```python
from build123d import *

# Parameters (mm, degrees)
F0_R     = 1.5875
F1_DEPTH = 12.7
F2_W     = 4.18922
F2_H     = 3.175
F3_DEPTH = 1.5875
F4_W     = 3.647596
F4_H     = 5.093468
F4_H_2   = 3.670235
F5_DEPTH = 25.4


with BuildPart() as f1:
    # F0 (on Right) → F1 (new body, symmetric)
    with BuildSketch(Plane.YZ):
        Circle(F0_R)
    extrude(amount=F1_DEPTH, both=True)

    # F2 (on face) → F3 (join)
    with BuildSketch(Plane(origin=(-12.7, 0, 0), x_dir=(0, -1, 0), z_dir=(-1, 0, 0))):
        with Locations((-2.09461, 0)):
            Rectangle(F2_W, F2_H)
    extrude(amount=F3_DEPTH)

    # F4 (on face) → F5 (cut)
    with BuildSketch(Plane.XY.offset(1.5875)):
        with BuildLine():
            ThreePointArc((10.658555, 1.5875), (9.327825, -0.125735), (7.724933, -1.5875))
            Line((7.724933, -1.5875), (12.7, -1.5875))
            Line((12.7, -1.5875), (12.7, 1.5875))
            Line((12.7, 1.5875), (10.658555, 1.5875))
        make_face()
        with Locations((-13.995515, -0.959234)):
            Rectangle(F4_W, F4_H)
        with Locations((-13.995515, 3.422617)):
            Rectangle(F4_W, F4_H_2)
    extrude(amount=-F5_DEPTH, mode=Mode.SUBTRACT)


solid = f1.part
```
Can you work these out from the model? Positions are in its coordinate system, mm. Give positions to 0.01 mm unless a question says otherwise; leave off trailing zeros. Loops run counter-clockwise (first coordinate to the right, second up) from the corner with the lowest first, then second, coordinate; pieces in that order, holes last. Notation, with made-up numbers: M 69.5,81.25 L 76.5,81.25 A15 cw 76.5,104.25 Z; hole C 3,65.5 d3. An arc over 180 degrees is marked long. Use CSV: the item, a comma, the result in double quotes. Start each with the question number.
1. Imagine slicing it at A-A, the plane x = 0.25. Write out the boundary of the cut face in (y, z) (1 decimal), plus the area to 3 significant figures.
2. If I drill on L1, parallel to Y at x = -3.5, z = 0.1; L2, parallel to Y at x = 6.75, z = -1.1; L3, parallel to Z at x = -10.25, y = 0.6, over which ranges is the centre line in solid material (lowest first)?
3. Imagine slicing it at B-B, the plane z = 0. Write out the boundary of the cut face in (x, y), plus the area to 3 significant figures.
4. Imagine slicing it at C-C, the plane y = -0.4. Write out the boundary of the cut face in (x, z).
5. For P1, Ø1.5, axis at x = -2, y = 1, coming from the +Z side; P2, Ø1, axis at x = -1, z = 1, coming from the +Y side, each with a flat end and sliding along its axis, tell me the tip position at first contact or that it passes through.
Response values:
1,outline,"C 0,0 d3.2"
1,area,"7.92 mm^2"
2,L1,"-1.58 to 1.58"
2,L2,"-1.14 to 1.14"
2,L3,"-1.47 to 1.47"
3,outline,"M -12.17,-1.59 L 7.72,-1.59 A12.7 ccw 10.66,1.59 L -12.17,1.59 Z"
3,area,"68.4 mm^2"
4,outline,"M -12.17,-1.54 L 9.07,-1.54 L 9.07,1.54 L -12.17,1.54 Z"
5,P1,"z = 1.57"
5,P2,"y = 1.51"
